```python
from build123d import *

# Parameters (mm, degrees)
BOSS_EXTRUDE1_DEPTH    = 1.5875
F_10_CLEARANCE_HOLE1_D = 4.9784
SKETCH5_R              = 14.057169334
CUT_EXTRUDE1_DEPTH     = 2.54


with BuildPart() as part:
    # Sketch2 → Boss-Extrude1 (new body)
    with BuildSketch(Plane(origin=(0, 0, 375.973880443), x_dir=(-1, 0, 0), z_dir=(0, 0, -1))):
        Polygon((-54.523488721, -26.582274219), (-27.603590087, -69.663117497), (-14.140826563, -61.250649173), (87.851311274, -224.47218895), (130.932154551, -197.552290315), (2.020118081, 8.750092739), align=None)
    extrude(amount=BOSS_EXTRUDE1_DEPTH)

    # #10 Clearance Hole1 (through all)
    with Locations(Plane(origin=(0, 0, 374.386380443), x_dir=(-1, 0, 0), z_dir=(0, 0, -1))):
        with Locations((-5.390733824, -63.270767254), (-25.583472007, -60.913024757), (-40.388290572, -25.23740497), (0, 0), (20.189923976, -32.310632459), (26.919898634, -43.080843278), (60.403864812, -96.66639049), (28.093232354, -116.856314466)):
            Hole(F_10_CLEARANCE_HOLE1_D / 2)

    # Sketch5 → Cut-Extrude1 (cut)
    with BuildSketch(Plane.XY.offset(375.973880443)):
        with Locations((19.523118196, -34.66274681)):
            Circle(SKETCH5_R)
    extrude(amount=-CUT_EXTRUDE1_DEPTH, mode=Mode.SUBTRACT)


solid = part.part
```
Geometry check sheet. Reference: the model listing, model coordinates, mm. A direction names the side the tool comes from. Round coordinates to 2 decimals unless told otherwise and drop trailing zeros. Loops run counter-clockwise (first coordinate to the right, second up) from the corner with the lowest first, then second, coordinate; pieces in that order, holes last. Notation, with made-up numbers: M -11,-18 L 21,-18 A35 ccw 21,21 Z; hole C -6,14 d9. An arc over 180 degrees is marked long. Return JSON: item names as keys, results as strings. Group by question number.
(1) Scan lines: line 1 along X through (y, z) = (-33.5, 375.5); line 2 along X through (y, z) = (-32.5, 375.2); line 3 along Y through (x, z) = (-19.5, 374.5). Record each from-to range of solid material in increasing order. Write a range as [from, to].
(2) Set-up check for faces 1 (the face through (42.763, -24.49, 375.191)), 2 (the face through (20.97, -65.52, 375.19)): record each of +Z, -Z, +X, -X, +Y, -Y from which the full face is reachable in a straight line by a thin tool's end or side.
(3) Section check B-B, the plane z = 374.85. Give the number of separate pieces and of enclosed holes in the cut face, and give its area (3 significant figures).
(4) Section check A-A, the plane y = 0. Enter the section's corners in (x, z), and give its area (3 significant figures).
(5) Section check D-D, the plane y = -148. Enter the section's corners in (x, z).
(6) Section check C-C, the plane x = -69. Enter the section's corners in (y, z), and give its area (3 significant figures).
(7) Go/stop test with a flat-tipped pin: pin 1 (6.5 mm diameter, centred on x = -28.09, y = -116.86, fed in from +Z). Record where the tip stops, or that it passes through.
(8) Mould release check, pull along X, two halves, no side actions. Record for faces 3 (the face through (-45, -116, 375.974)), 4 (the face through (25.259, -58.445, 375.191)), 5 (the face through (-109.09, -211.2, 375.19)): pulls with the +X half, pulls with the -X half, needs draft (parallel to the pull), parting line crosses it, or undercut.
Data:
{
 "1": {"line 1": "[-28.42, -22.38], [-18, 5.51], [33.53, 50.2]", "line 2": "[-27.8, -22.67], [-17.71, 5.63], [33.41, 50.83]", "line 3": "[-115.09, -34.7], [-29.92, -19.22]"},
 "2": {"face 1": "+Z, -Z", "face 2": "+Z, -Z, -Y"},
 "3": {"separate pieces": "1", "enclosed holes": "9", "area": "12,400 mm²"},
 "4": {"outline": "M -7.49,374.39 L -2.49,374.39 L -2.49,375.97 L -7.49,375.97 Z; M 2.49,374.39 L 11.98,374.39 L 11.98,375.97 L 2.49,375.97 Z", "area": "23.0 mm²"},
 "5": {"outline": "M -99.97,374.39 L -40.07,374.39 L -40.07,375.97 L -99.97,375.97 Z"},
 "6": {"outline": "M -194.3,374.39 L -98.44,374.39 L -98.44,375.97 L -194.3,375.97 Z", "area": "152 mm²"},
 "7": {"pin 1": "z = 375.97"},
 "8": {"face 3": "needs draft", "face 4": "undercut", "face 5": "pulls with the -X half"}
}
